The listing builds one solid part. Answer for the finished solid, in the listing's coordinates (mm). A direction names the side the tool comes from. Coordinates: 2 decimals unless noted, no trailing zeros. Loops run counter-clockwise (first coordinate to the right, second up) from the corner with the lowest first, then second, coordinate; pieces in that order, holes last. Notation, with made-up numbers: M -25.75,-28 L 3.25,-28 A17 ccw 3.25,-1 Z; hole C -15.75,-1.75 d10. An arc over 180 degrees is marked long. Return JSON: item names as keys, results as strings. Group by question number.
1. Section C-C (z = -1.5) is taken. Write down the section's boundary in (x, y).
2. Given P1, Ø5, axis at x = 17.5, z = -11, coming from the -Y side; P2, Ø8, axis at y = 12.5, z = -2.5, coming from the -X side (3 decimals); P3, Ø6.5, axis at x = 21.5, z = -6.5, coming from the +Y side, each flat-ended and moving along its own axis, determine where each tip first touches the part or whether it passes through.
3. Section A-A (y = 42.5) is taken. Write down the section's boundary in (x, z) (3 decimals).
4. Straight lines are drawn through the part: L1, parallel to Y at x = 27.5, z = -4.75; L2, parallel to Z at x = 44.5, y = 40.5 (3 decimals). For each, find the intervals that lie inside material, in ascending order. Write a range as from..to.
5. Which of the six approach directions +Z, -Z, +X, -X, +Y, -Y give full straight-line access (tool end or side, diameter ignored) to faces 1 (the face through (0, 22, -6)), 2 (the face through (44.45, 22, -6)), 3 (the face through (22, 0, -6))?
```python
from build123d import *

# Parameters (mm, degrees)
SKETCH1_W           = 50.8
SKETCH1_H           = 50.8
SKETCH1_W_2         = 44.45
SKETCH1_H_2         = 44.45
BOSS_EXTRUDE1_DEPTH = 3.175
SKETCH1_4_W         = 44.45
SKETCH1_4_H         = 44.45
BOSS_EXTRUDE2_DEPTH = 12.7


with BuildPart() as part:
    # Sketch1 → Boss-Extrude1 (new body)
    with BuildSketch(Plane.XY):
        with Locations((22.225, 22.225)):
            Rectangle(SKETCH1_W, SKETCH1_H)
        with Locations((22.225, 22.225)):
            Rectangle(SKETCH1_W_2, SKETCH1_H_2, mode=Mode.SUBTRACT)
        with Locations((22.225, 22.225)):
            Rectangle(SKETCH1_W_2, SKETCH1_H_2)
    extrude(amount=BOSS_EXTRUDE1_DEPTH)

    # Sketch1_4 → Boss-Extrude2 (add)
    with BuildSketch(Plane.XY):
        with Locations((22.225, 22.225)):
            Rectangle(SKETCH1_4_W, SKETCH1_4_H)
    extrude(amount=-BOSS_EXTRUDE2_DEPTH)


solid = part.part
```
Worked out:
{
 "1": {"outline": "M 0,0 L 44.45,0 L 44.45,44.45 L 0,44.45 Z"},
 "2": {"P1": "y = 0", "P2": "x = -3.175", "P3": "y = 44.45"},
 "3": {"outline": "M -3.175,0 L 0,0 L 0,-12.7 L 44.45,-12.7 L 44.45,0 L 47.625,0 L 47.625,3.175 L -3.175,3.175 Z"},
 "4": {"L1": "0..44.45", "L2": "0..3.175"},
 "5": {"face 1": "-Z, -X, +Y, -Y", "face 2": "-Z, +X, +Y, -Y", "face 3": "-Z, +X, -X, -Y"}
}
